Part model, mm, in its own coordinate system. A direction names the side the tool comes from. Coordinates: 2 decimals unless noted, no trailing zeros. Loops run counter-clockwise (first coordinate to the right, second up) from the corner with the lowest first, then second, coordinate; pieces in that order, holes last. Notation, with made-up numbers: (-21, 72.25) - (0, 72.25) arc R24 ccw to (0, 98.25) - close; hole circle Ø8 at (49.25, 78.25). An arc over 180 degrees is marked (long way). Answer as CSV lines item,"result".
from build123d import *

# Parameters (mm, degrees)
BOSS_EXTRUDE1_DEPTH  = 10
SKETCH2_W            = 10.336230878
SKETCH2_H            = 10.881732654
SKETCH2_W_2          = 8
SKETCH2_H_2          = 9
BOSS_EXTRUDE2_DEPTH  = 10
EXTRUDE_THIN1_DEPTH  = 30
BOSS_EXTRUDE3_DEPTH  = 1
MIRROR2_COPY_1_DEPTH = 1
CHAMFER2_SIZE        = 3
CUT_EXTRUDE1_DEPTH   = 5


with BuildPart() as part:
    # Sketch1 → Boss-Extrude1 (new body)
    with BuildSketch(Plane.XY):
        Polygon((0, 14.392304845), (-12.464101615, -7.196152423), (12.464101615, -7.196152423), align=None)
        Polygon((0, 10.392304845), (-9, -5.196152423), (9, -5.196152423), align=None, mode=Mode.SUBTRACT)
    extrude(amount=BOSS_EXTRUDE1_DEPTH)

    # Sketch2 → Boss-Extrude2 (add)
    with BuildSketch(Plane.XY.offset(10)):
        Rectangle(SKETCH2_W, SKETCH2_H)
        Rectangle(SKETCH2_W_2, SKETCH2_H_2, mode=Mode.SUBTRACT)
    extrude(amount=-BOSS_EXTRUDE2_DEPTH)

    # Sketch3 → Extrude-Thin1 (add)
    with BuildSketch(Plane.XY.offset(10)):
        Polygon((0, 14.392304845), (-12.464101615, -7.196152423), (12.464101615, -7.196152423), align=None)
        Polygon((0, 12.392304845), (-10.732050808, -6.196152423), (10.732050808, -6.196152423), align=None, mode=Mode.SUBTRACT)
    extrude(amount=EXTRUDE_THIN1_DEPTH)

    # Sketch4 → Boss-Extrude3 (add, symmetric)
    with BuildSketch(Plane(origin=(0, 0, 0), x_dir=(0.866025404, 0.5, 0), z_dir=(-0.5, 0.866025404, 0))):
        Polygon((7.196152423, -2.618036355), (7.196152423, -14.298247708), (15.718557778, -19.278268119), (20.919199073, -32.180049847), (18.151461796, -61.156795565), (25.431971062, -28.309033375), (18.151461796, -10.247502864), align=None)
    boss_extrude3 = extrude(amount=BOSS_EXTRUDE3_DEPTH, both=True)

    # Mirror1: Boss-Extrude3 across plane
    add(boss_extrude3.mirror(Plane(origin=(0, 0, 0), x_dir=(0, 0, 1), z_dir=(1, 0, 0))))

    # Mirror2: Boss-Extrude3 across plane
    add(boss_extrude3.mirror(Plane(origin=(0, 0, 0), x_dir=(0, 0, 1), z_dir=(-0.5, 0.866025404, 0))))

    # Mirror2 copy 1 sketch → Mirror2 copy 1 (add, symmetric)
    with BuildSketch(Plane(origin=(0, 0, 0), x_dir=(0, -1, 0), z_dir=(1, 0, 0))):
        Polygon((7.196152423, -2.618036355), (7.196152423, -14.298247708), (15.718557778, -19.278268119), (20.919199073, -32.180049847), (18.151461796, -61.156795565), (25.431971062, -28.309033375), (18.151461796, -10.247502864), align=None)
    extrude(amount=MIRROR2_COPY_1_DEPTH, both=True)

    # Chamfer2
    chamfer2_edges = [part.edges().sort_by_distance(p)[0] for p in [
        (6.732050808, 2.732050808, 8.458142032),
        (5.732050808, 4.464101615, 8.458142032),
        (-5.732050808, 4.464101615, 8.458142032),
        (-6.732050808, 2.732050808, 8.458142032),
        (-1, -7.196152423, 8.458142032),
        (1, -7.196152423, 8.458142032),
    ]]
    chamfer(chamfer2_edges, length=CHAMFER2_SIZE)

    # Sketch5 → Cut-Extrude1 (cut)
    with BuildSketch(Plane(origin=(0, 0, 0), x_dir=(-1, 0, 0), z_dir=(0, 0, -1))):
        Polygon((0, 10.392304845), (-9, -5.196152423), (9, -5.196152423), align=None)
    extrude(amount=-CUT_EXTRUDE1_DEPTH, mode=Mode.SUBTRACT)


solid = part.part
Q1. Wall check: L1, parallel to X at y = 2, z = 23; L2, parallel to Z at x = -3.5, y = 6.5; L3, parallel to Y at x = 7.5, z = 29.5. Give the ranges that are in metal, low to high.
Results:
L1,"x = -7.15 to -6, 6 to 7.15"
L2,"z = 0 to 40"
L3,"y = -7.2 to -6.2, -0.6 to 1.4"
Q2. Saw through at B-B (x = 2). Give the cut face in (y, z).
Results:
outline,"(-9.2, 4.01) - (-7.2, 2.62) - (-7.2, 0) - (-5.2, 0) - (-5.2, 5) - (-4.5, 5) - (-4.5, 10) - (-6.2, 10) - (-6.2, 40) - (-7.2, 40) - (-7.2, 14.3) - (-9.2, 15.47) - close; (4.5, 5) - (5.44, 5) - (5.44, 10) - (4.5, 10) - close; (6.93, 0) - (10.93, 0) - (10.93, 40) - (8.93, 40) - (8.93, 10) - (6.93, 10) - close"
Q3. Saw through at D-D (x = -11.5). Give the cut face in (y, z).
Results:
outline,"(-7.2, 0) - (-5.53, 0) - (-5.53, 40) - (-7.2, 40) - close; (5.48, 6.45) - (7.79, 7.26) - (7.79, 18.19) - (5.48, 17.52) - close"
Q4. Saw through at A-A (z = 30). Give the cut face in (x, y), then the cut area to 3 significant figures.
Results:
outline,"(-22.2, 11.66) - (-17.86, 9.15) - (-16.86, 10.89) - (-21.2, 13.39) - close; (-12.46, -7.2) - (12.46, -7.2) - (0, 14.39) - close; (-1, -25.06) - (1, -25.06) - (1, -20.04) - (-1, -20.04) - close; (16.86, 10.89) - (17.86, 9.15) - (22.2, 11.66) - (21.2, 13.39) - close; hole (-10.73, -6.2) - (10.73, -6.2) - (0, 12.39) - close"
area,"99.7 mm^2"
Q5. Saw through at C-C (z = 53). Give the cut face in (x, y).
Results:
outline,"(-17.79, 9.11) - (-16.89, 8.6) - (-15.89, 10.33) - (-16.79, 10.85) - close; (-1, -19.96) - (1, -19.96) - (1, -18.93) - (-1, -18.93) - close; (15.89, 10.33) - (16.89, 8.6) - (17.79, 9.11) - (16.79, 10.85) - close"
Q6. Flat gauge pins, fed straight in: pin 1 (3 mm diameter, centred on x = -14, z = 31.5, fed in from -Y); pin 2 (2.5 mm diameter, centred on x = 0.5, z = 8, fed in from +Y); pin 3 (3 mm diameter, centred on x = 3, z = 4, fed in from +Y); pin 4 (1.5 mm diameter, centred on x = 3.5, y = -3, fed in from +Z). Where does each tip first touch, or does it go through?
Results:
pin 1,"passes through"
pin 2,"stops at y = 14.39"
pin 3,"stops at y = 11.79"
pin 4,"stops at z = 10"
Q7. Two-plate mould, pull along Z, no slides. Class faces 1 (the face through (0, -5, 5)), 2 (the face through (2.479, -8.717, 9.241)), 3 (the face through (-15.83, 9.15, 25.64)): released by +Z, released by -Z, zero draft, split by the parting line, or undercut.
Results:
face 1,"released by -Z"
face 2,"zero draft"
face 3,"undercut"
Q8. Which spindle directions (+Z, -Z, +X, -X, +Y, -Y) get a long thin tool onto all of the face, cutting with end or side? Do faces 4 (the face through (16.928, 9.789, 46.466)), 5 (the face through (16.874, 8.588, 22.347)), 6 (the face through (1, -19, 22)). Say none if no direction does.
Results:
face 4,"-Y"
face 5,"+Z, -Z, +X"
face 6,"+Z, -Z, +X, -Y"
